```python
from build123d import *

# Parameters (mm, degrees)
F1_DEPTH  = 395.5
F2_R      = 20
F3_DEPTH  = 70.001
F4_W      = 5
F4_H      = 122
F5_DEPTH  = 5
F6_R      = 6.5
F7_DEPTH  = 75.001
F8_SIZE   = 5
F11_DEPTH = 175.001


with BuildPart() as f1:
    # F0 (on Top) → F1 (new body, symmetric)
    with BuildSketch(Plane.XY):
        with BuildLine():
            Line((-85, 57), (-85, 0))
            Line((-85, 0), (-80, 0))
            Line((-80, 0), (-80, 57))
            ThreePointArc((-80, 57), (-77.6568542495, 62.6568542495), (-72, 65))
            Line((-72, 65), (72, 65))
            ThreePointArc((72, 65), (77.6568542495, 62.6568542495), (80, 57))
            Line((80, 57), (80, 0))
            Line((80, 0), (85, 0))
            Line((85, 0), (85, 57))
            ThreePointArc((85, 57), (81.1923881554, 66.1923881554), (72, 70))
            Line((72, 70), (-72, 70))
            ThreePointArc((-72, 70), (-81.1923881554, 66.1923881554), (-85, 57))
        make_face()
    extrude(amount=F1_DEPTH, both=True)

    # F2 (on face) → F3 (cut, through all)
    with BuildSketch(Plane(origin=(0, 70, 0), x_dir=(-1, 0, 0), z_dir=(0, 1, 0))):
        with Locations((0, -323.5)):
            Circle(F2_R)
        with BuildLine():
            Line((-47.5, -102.5), (-62.5, -102.5))
            ThreePointArc((-62.5, -102.5), (-68, -108), (-62.5, -113.5))
            Line((-62.5, -113.5), (-47.5, -113.5))
            ThreePointArc((-47.5, -113.5), (-42, -108), (-47.5, -102.5))
        make_face()
        with Locations((0, 323.5)):
            Circle(F2_R)
        with BuildLine():
            Line((-47.5, 237.5), (-62.5, 237.5))
            ThreePointArc((-62.5, 237.5), (-68, 232), (-62.5, 226.5))
            Line((-62.5, 226.5), (-47.5, 226.5))
            ThreePointArc((-47.5, 226.5), (-42, 232), (-47.5, 237.5))
        make_face()
        with BuildLine():
            Line((47.5, 226.5), (62.5, 226.5))
            ThreePointArc((62.5, 226.5), (68, 232), (62.5, 237.5))
            Line((62.5, 237.5), (47.5, 237.5))
            ThreePointArc((47.5, 237.5), (42, 232), (47.5, 226.5))
        make_face()
        with BuildLine():
            ThreePointArc((62.5, -113.5), (68, -108), (62.5, -102.5))
            Line((62.5, -102.5), (47.5, -102.5))
            ThreePointArc((47.5, -102.5), (42, -108), (47.5, -113.5))
            Line((47.5, -113.5), (62.5, -113.5))
        make_face()
    extrude(amount=-F3_DEPTH, mode=Mode.SUBTRACT)



with BuildPart() as f5:
    # F4 (on face) → F5 (new body)
    with BuildSketch(Plane.XZ):
        Polygon((-90, -273.5), (-90, -403.5), (90, -403.5), (90, -273.5), (-80, -273.5), (-80, -395.5), (-85, -395.5), (-85, -273.5), align=None)
        with Locations((-82.5, -334.5)):
            Rectangle(F4_W, F4_H)
    extrude(amount=F5_DEPTH)

    # F6 (on face) → F7 (cut, through all)
    with BuildSketch(Plane.XZ.offset(5)):
        with Locations((0, -323.5)):
            Circle(F6_R)
    extrude(amount=-F7_DEPTH, mode=Mode.SUBTRACT)

    # F8
    f8_edges = [f5.edges().sort_by_distance(p)[0] for p in [
        (-90, -2.5, -273.5),
        (90, -2.5, -273.5),
        (-90, -2.5, -403.5),
        (90, -2.5, -403.5),
    ]]
    chamfer(f8_edges, length=F8_SIZE)


with BuildPart() as f1_1:
    add(f1.part)

    add(f5.part)  # F9 merges F5
    # F9: F5 across plane
    add(f5.part.mirror(Plane.XY))

    # F10 (on face) → F11 (cut, through all)
    with BuildSketch(Plane(origin=(-85, 0, 0), x_dir=(0, -1, 0), z_dir=(-1, 0, 0))):
        Polygon((-70, -395.5), (-57, -395.5), (-57, -348.5), (-70, -335.5), align=None)
        Polygon((-57, -395.5), (-10, -395.5), (-57, -348.5), align=None)
        Polygon((-70, 335.5), (-57, 348.5), (-57, 395.5), (-70, 395.5), align=None)
        Polygon((-57, 395.5), (-57, 348.5), (-10, 395.5), align=None)
    extrude(amount=-F11_DEPTH, mode=Mode.SUBTRACT)


solid = f1_1.part
```
Verification items for the finished model (mm, model axes). A direction names the side the tool comes from. Round coordinates to 2 decimals unless told otherwise and drop trailing zeros. Write each loop counter-clockwise with the first axis right and the second up, starting at its lowest first coordinate (ties: lowest second). Pieces come first, ordered by that corner, then holes. Notation, with made-up numbers: (24.5, 30.5) - (43.5, 30.5) arc R32 cw to (43.5, 61.5) - close; hole circle Ø7 at (-28, 67). An arc over 180 degrees is marked (long way). Answer as a JSON object with one key per item and string values. Group by question number.
Q1. Thickness scan on line 1 (Z direction, x = 0, y = -1); line 2 (X direction, y = -3, z = -323); line 3 (X direction, y = 14.5, z = 41). Record the ranges inside material, lowest first.
Q2. Tool access check on faces 1 (the cylindrical face through (0.724, 67.535, 303.513)), 2 (the flat face through (85, 28, 6)), 3 (the flat face through (-80, 28, 6)). Record the directions out of +Z, -Z, +X, -X, +Y, -Y that give a thin tool (end or side, any length) a straight path to the whole face; none if there is none.
Q3. Go/stop test with flat-tipped pins: pin 1 Ø3 at (y, z) = (28.5, -158.5) entering from -X; pin 2 Ø1.5 at (x, y) = (52.5, 67.5) entering from -Z; pin 3 Ø4 at (x, y) = (82, 7) entering from -Z. Record where each tip stops, or that it passes through.
Q4. Section check A-A, the plane y = 21.5. Enter the section's corners in (x, z), plus the area to 3 significant figures.
Q5. Mould release check, pull along Y, two halves, no side actions. Record for faces 4 (the cylindrical face through (81.293, 66.091, 4.879)), 5 (the flat face through (19, 0, 338)), 6 (the flat face through (-1, 65, 5)), 7 (the cylindrical face through (3.494, -2.535, 318.019)): released by +Y, released by -Y, zero draft, split by the parting line, or undercut.
Q6. Section check B-B, the plane z = 39. Enter the section's corners in (x, y).
Found:
{
 "1": {"line 1": "z = -403.5 to -330, -317 to -273.5, 273.5 to 317, 330 to 403.5", "line 2": "x = -90 to -6.48, 6.48 to 90", "line 3": "x = -85 to -80, 80 to 85"},
 "2": {"face 1": "+Y", "face 2": "+Z, -Z, +X, +Y", "face 3": "+Z, -Z"},
 "3": {"pin 1": "stops at x = -85", "pin 2": "stops at z = -338.75", "pin 3": "stops at z = -395.5"},
 "4": {"outline": "(-85, -384) - (-80, -384) - (-80, 384) - (-85, 384) - close; (80, -384) - (85, -384) - (85, 384) - (80, 384) - close", "area": "7,680 mm^2"},
 "5": {"face 4": "released by +Y", "face 5": "undercut", "face 6": "undercut", "face 7": "zero draft"},
 "6": {"outline": "(-85, 0) - (-80, 0) - (-80, 57) arc R8 cw to (-72, 65) - (72, 65) arc R8 cw to (80, 57) - (80, 0) - (85, 0) - (85, 57) arc R13 ccw to (72, 70) - (-72, 70) arc R13 ccw to (-85, 57) - close"}
}
